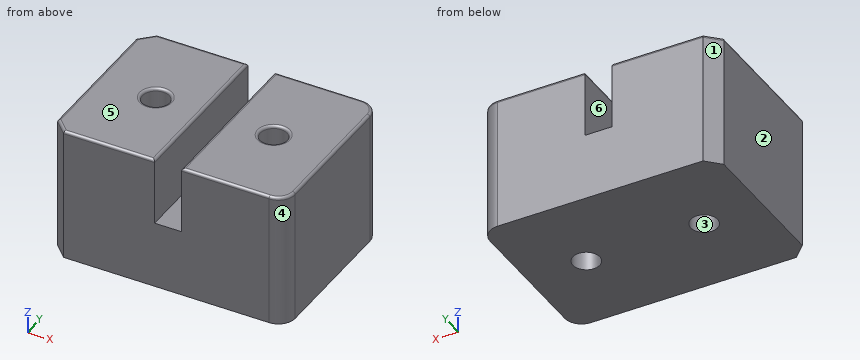
```python
from build123d import *

# Parameters (mm, degrees)
SKETCH_W     = 70
SKETCH_H     = 50
SKETCH_R     = 4
PAD_DEPTH    = 40
SKETCH001_W  = 8
SKETCH001_H  = 50
POCKET_DEPTH = 20
FILLET_R     = 5
CHAMFER_SIZE = 4
FILLET001_R  = 0.8
FILLET002_R  = 0.8


with BuildPart() as part:
    # Sketch → Pad (new body)
    with BuildSketch(Plane.XY):
        with Locations((35, 25)):
            Rectangle(SKETCH_W, SKETCH_H)
        with Locations((17.5, 25)):
            Circle(SKETCH_R, mode=Mode.SUBTRACT)
        with Locations((52.5, 25)):
            Circle(SKETCH_R, mode=Mode.SUBTRACT)
    extrude(amount=PAD_DEPTH)

    # Sketch001 (on Face8 of Pad) → Pocket (cut)
    with BuildSketch(Plane.XY.offset(40)):
        with Locations((35, 25)):
            Rectangle(SKETCH001_W, SKETCH001_H)
    extrude(amount=-POCKET_DEPTH, mode=Mode.SUBTRACT)

    # Fillet
    fillet_edges = [part.edges().sort_by_distance(p)[0] for p in [
        (70, 0, 20),
        (70, 50, 20),
    ]]
    fillet(fillet_edges, radius=FILLET_R)

    # Chamfer
    chamfer_edges = [part.edges().sort_by_distance(p)[0] for p in [
        (0, 50, 20),
        (0, 0, 20),
    ]]
    chamfer(chamfer_edges, length=CHAMFER_SIZE)

    # Fillet001
    fillet001_edges = [part.edges().sort_by_distance(p)[0] for p in [
        (52, 50, 40),
        (68.535534, 48.535534, 40),
        (39, 25, 40),
        (70, 25, 40),
        (52, 0, 40),
        (68.535534, 1.464466, 40),
        (48.5, 25, 40),
    ]]
    fillet(fillet001_edges, radius=FILLET001_R)

    # Fillet002
    fillet002_edges = [part.edges().sort_by_distance(p)[0] for p in [
        (17.5, 50, 40),
        (2, 48, 40),
        (31, 25, 40),
        (0, 25, 40),
        (17.5, 0, 40),
        (2, 2, 40),
        (13.5, 25, 40),
    ]]
    fillet(fillet002_edges, radius=FILLET002_R)


solid = part.part
```
Build history of the part. All positions in model axes, mm. Face numbers are marked on the shaded views. A direction names the side the tool comes from. Coordinates: 2 decimals unless noted, no trailing zeros. Order: outer loops, then holes, each group sorted by start corner. A loop starts at its lowest first (then second) coordinate and runs counter-clockwise, first axis right, second up.
Item 1: Saw through at D-D on z = 17.5. List the corners of the cut face in (x, y).
Filled in:
outline: (0, 4) - (4, 0) - (65, 0) arc R5 ccw to (70, 5) - (70, 45) arc R5 ccw to (65, 50) - (4, 50) - (0, 46) - close; hole circle Ø8 at (17.5, 25); hole circle Ø8 at (52.5, 25)
Item 2: Mould opens along Y. For the marked faces 1, 2, 3 and 4 say: released by +Y, released by -Y, zero draft, split by the parting line, or undercut.
Filled in:
face 1: released by +Y
face 2: zero draft
face 3: undercut
face 4: released by -Y
Item 3: Tool access for the marked faces 5 and 6: list every direction of +Z, -Z, +X, -X, +Y, -Y with a clear straight run to the whole face (end or side of a thin tool).
Filled in:
face 5: +Z, +X, -X, +Y, -Y
face 6: +Z, +Y, -Y
Item 4: Saw through at B-B on x = 17.5. List the corners of the cut face in (y, z), then the cut area to 3 significant figures.
Filled in:
outline: (0, 0) - (21, 0) - (21, 39.2) arc R0.8 ccw to (20.2, 40) - (0.8, 40) arc R0.8 ccw to (0, 39.2) - close; (29, 0) - (50, 0) - (50, 39.2) arc R0.8 ccw to (49.2, 40) - (29.8, 40) arc R0.8 ccw to (29, 39.2) - close
area: 1,680 mm2
Item 5: Drill centre lines: L1, parallel to X at y = 45, z = 28.5; L2, parallel to Z at x = 34.5, y = 23; L3, parallel to Y at x = 17.5, z = 28.5. Where is each one in solid material? Low to high.
Filled in:
L1: x = 0 to 31, 39 to 70
L2: z = 0 to 20
L3: y = 0 to 21, 29 to 50
Item 6: Saw through at A-A on z = 30. List the corners of the cut face in (x, y), then the cut area to 3 significant figures.
Filled in:
outline: (0, 4) - (4, 0) - (31, 0) - (31, 50) - (4, 50) - (0, 46) - close; (39, 0) - (65, 0) arc R5 ccw to (70, 5) - (70, 45) arc R5 ccw to (65, 50) - (39, 50) - close; hole circle Ø8 at (17.5, 25); hole circle Ø8 at (52.5, 25)
area: 2,970 mm2
Item 7: Drop flat-ended pins along their axis: pin 1 Ø13 at (x, y) = (52.5, 25) entering from +Z; pin 2 Ø1 at (x, y) = (31, 42.5) entering from +Z. Give the stop position or say it passes through.
Filled in:
pin 1: stops at z = 40
pin 2: stops at z = 39.94
Item 8: Saw through at C-C on y = 25. List the corners of the cut face in (x, z), then the cut area to 3 significant figures.
Filled in:
outline: (0, 0) - (13.5, 0) - (13.5, 39.2) arc R0.8 ccw to (12.7, 40) - (0.8, 40) arc R0.8 ccw to (0, 39.2) - close; (21.5, 0) - (48.5, 0) - (48.5, 39.2) arc R0.8 ccw to (47.7, 40) - (39.8, 40) arc R0.8 ccw to (39, 39.2) - (39, 20) - (31, 20) - (31, 39.2) arc R0.8 ccw to (30.2, 40) - (22.3, 40) arc R0.8 ccw to (21.5, 39.2) - close; (56.5, 0) - (70, 0) - (70, 39.2) arc R0.8 ccw to (69.2, 40) - (57.3, 40) arc R0.8 ccw to (56.5, 39.2) - close
area: 2,000 mm2
